from build123d import *

# Parameters (mm, degrees)
BOSS_EXTRUDE1_DEPTH     = 25.4
SKETCH2_R               = 3.175
BOSS_EXTRUDE3_DEPTH     = 3.81
BOSS_EXTRUDE4_START     = 3.81
SKETCH3_R               = 3.175
BOSS_EXTRUDE4_DEPTH     = 3.81
SKETCH4_W               = 19.976191583
SKETCH4_H               = 93.98
BOSS_EXTRUDE5_DEPTH     = 5.08
CUT_EXTRUDE1_DEPTH      = 5.08
CUT_EXTRUDE1_DEPTH_BACK = 381.820097899
SKETCH5_R               = 3.175


with BuildPart() as part:
    # Sketch1 → Boss-Extrude1 (new body)
    with BuildSketch(Plane.XY):
        with BuildLine():
            Line((-348.791316574, 206.904032246), (-347.931840304, 210.615824339))
            Line((-347.931840304, 210.615824339), (-357.71784023, 212.881801123))
            ThreePointArc((-357.71784023, 212.881801123), (-360.881852793, 214.462416261), (-362.982664296, 217.307747657))
            ThreePointArc((-362.982664296, 217.307747657), (-363.332122594, 222.183147168), (-360.629697113, 226.256050065))
            ThreePointArc((-360.629697113, 226.256050065), (-361.446766946, 231.453900041), (-358.789055407, 235.995025106))
            Line((-358.789055407, 235.995025106), (-363.476973871, 237.08052628))
            Line((-363.476973871, 237.08052628), (-369.361521397, 211.667123083))
            Line((-369.361521397, 211.667123083), (-348.791316574, 206.904032246))
        make_face()
    extrude(amount=-BOSS_EXTRUDE1_DEPTH)

    # Sketch2 → Boss-Extrude3 (add)
    # profile 1 of 2: a face of its own
    with BuildSketch(Plane(origin=(0, 0, -25.4), x_dir=(-1, 0, 0), z_dir=(0, 0, -1))):
        with BuildLine():
            Line((342.906769048, 232.317435443), (358.789055407, 235.995025106))
            ThreePointArc((358.789055407, 235.995025106), (361.446766946, 231.453900041), (360.629697113, 226.256050065))
            ThreePointArc((360.629697113, 226.256050065), (363.40772554, 218.647103628), (357.71784023, 212.881801123))
            Line((357.71784023, 212.881801123), (347.931840304, 210.615824339))
            Line((347.931840304, 210.615824339), (342.906769048, 232.317435443))
        make_face()
        with Locations(Location((353.754071424, 230, 0), (0, 0, 180))):
            Circle(SKETCH2_R, mode=Mode.SUBTRACT)
        with Locations(Location((356.009914651, 220.257763535, 0), (0, 0, 180))):
            Circle(SKETCH2_R, mode=Mode.SUBTRACT)
    # profile 2 of 2: a face of its own
    with BuildSketch(Plane(origin=(0, 0, -25.4), x_dir=(-1, 0, 0), z_dir=(0, 0, -1))):
        with BuildLine():
            ThreePointArc((360.629697113, 226.256050065), (363.40772554, 218.647103628), (357.71784023, 212.881801123))
            Line((357.71784023, 212.881801123), (347.931840304, 210.615824339))
            Line((347.931840304, 210.615824339), (348.791316574, 206.904032246))
            Line((348.791316574, 206.904032246), (369.361521397, 211.667123083))
            Line((369.361521397, 211.667123083), (363.476973871, 237.08052628))
            Line((363.476973871, 237.08052628), (358.789055407, 235.995025106))
            ThreePointArc((358.789055407, 235.995025106), (361.446766946, 231.453900041), (360.629697113, 226.256050065))
        make_face()
    extrude(amount=BOSS_EXTRUDE3_DEPTH)

    # Sketch3 → Boss-Extrude4 (add)
    # profile 1 of 2: a face of its own
    with BuildSketch(Plane.XY.offset(BOSS_EXTRUDE4_START)):
        with BuildLine():
            Line((-342.906769048, 232.317435443), (-358.789055407, 235.995025106))
            ThreePointArc((-358.789055407, 235.995025106), (-361.446766946, 231.453900041), (-360.629697113, 226.256050065))
            ThreePointArc((-360.629697113, 226.256050065), (-363.40772554, 218.647103628), (-357.71784023, 212.881801123))
            Line((-357.71784023, 212.881801123), (-347.931840304, 210.615824339))
            Line((-347.931840304, 210.615824339), (-342.906769048, 232.317435443))
        make_face()
        with Locations((-356.009914651, 220.257763535)):
            Circle(SKETCH3_R, mode=Mode.SUBTRACT)
        with Locations((-353.754071424, 230)):
            Circle(SKETCH3_R, mode=Mode.SUBTRACT)
    # profile 2 of 2: a face of its own
    with BuildSketch(Plane.XY.offset(BOSS_EXTRUDE4_START)):
        with BuildLine():
            Line((-347.931840304, 210.615824339), (-357.71784023, 212.881801123))
            ThreePointArc((-357.71784023, 212.881801123), (-363.40772554, 218.647103628), (-360.629697113, 226.256050065))
            ThreePointArc((-360.629697113, 226.256050065), (-361.446766946, 231.453900041), (-358.789055407, 235.995025106))
            Line((-358.789055407, 235.995025106), (-363.476973871, 237.08052628))
            Line((-363.476973871, 237.08052628), (-369.361521397, 211.667123083))
            Line((-369.361521397, 211.667123083), (-348.791316574, 206.904032246))
            Line((-348.791316574, 206.904032246), (-347.931840304, 210.615824339))
        make_face()
    extrude(amount=-BOSS_EXTRUDE4_DEPTH)

    # Sketch4 → Boss-Extrude5 (add)
    with BuildSketch(Plane(origin=(0, 211.667123083, 0), x_dir=(1, 0, 0), z_dir=(0, 1, 0))):
        with Locations((-365.660654241, 10.16)):
            Rectangle(SKETCH4_W, SKETCH4_H)
    extrude(amount=-BOSS_EXTRUDE5_DEPTH)

    # Sketch5 → Cut-Extrude1 (cut, two sides: drawn at the far end of the back side and taken through both)
    with BuildSketch(Plane(origin=(0, 211.667123083, 0), x_dir=(1, 0, 0), z_dir=(0, 1, 0)).offset(-CUT_EXTRUDE1_DEPTH_BACK)):
        with Locations(Location((-366.758750033, 43.909082713, 0), (0, 0, 270))):
            Circle(SKETCH5_R)
        with Locations(Location((-366.758750033, -31.331908304, 0), (0, 0, 270))):
            Circle(SKETCH5_R)
    extrude(amount=CUT_EXTRUDE1_DEPTH + CUT_EXTRUDE1_DEPTH_BACK, mode=Mode.SUBTRACT)


solid = part.part
Can you work these out from the model? Positions are in its coordinate system, mm. A direction names the side the tool comes from. Round coordinates to 2 decimals unless told otherwise and drop trailing zeros. Loops run counter-clockwise (first coordinate to the right, second up) from the corner with the lowest first, then second, coordinate; pieces in that order, holes last. Notation, with made-up numbers: (45.5, 28) - (52.5, 28) arc R8 ccw to (52.5, 33) - close; hole circle Ø3 at (46, 74.25). An arc over 180 degrees is marked (long way). Use CSV: the item, a comma, the result in double quotes. Start each with the question number.
1) For faces 1 (the flat face through (-352.28, 207.71, -12.47)), 2 (the flat face through (-353, 223, -25.4)), 3 (the flat face through (-352.756, 211.733, -12.522)), which set-ups out of +Z, -Z, +X, -X, +Y, -Y let a thin tool reach every point of the face, with its end or its side?
2) If we section it at C-C on y = 235: Write out the boundary of the cut face in (x, z), plus the area to 3 significant figures.
3) If we section it at A-A on z = -10: Write out the boundary of the cut face in (x, y), plus the area to 3 significant figures.
4) If we section it at B-B on y = 219: Write out the boundary of the cut face in (x, z), plus the area to 3 significant figures.
5) For pin 1 Ø10 at (x, z) = (-366.76, 31.33) entering from +Y; pin 2 Ø13 at (x, y) = (-362, 216.5) entering from +Z; pin 3 Ø4 at (x, y) = (-353.75, 230) entering from -Z; pin 4 Ø16.5 at (x, y) = (-357.5, 222.5) entering from -Z, each with a flat end and sliding along its axis, tell me the tip position at first contact or that it passes through.
6) If we section it at D-D on y = 230: Write out the boundary of the cut face in (x, z).
7) We'd pull the mould along X, two halves only. Please class faces 4 (the flat face through (-353, 222, 3.81)), 5 (the flat face through (-375.649, 209, -10)), 6 (the cylindrical face through (-369.858, 209.092, 30.644)): released by +X, released by -X, zero draft, split by the parting line, or undercut.
8) Please list where these lines run through material, in increasing order: probe 1 along Y at (x, z) = (-353.5, 1); probe 2 along Z at (x, y) = (-365.5, 208.5); probe 3 along Z at (x, y) = (-358, 233.5). Write a range as [from, to].
Geometry results:
1,face 1,"+Z, -Z, -Y"
1,face 2,"+X"
1,face 3,"+X, +Y"
2,outline,"(-363.96, -29.21) - (-354.49, -29.21) - (-354.49, -25.4) - (-359.78, -25.4) - (-359.78, 0) - (-354.49, 0) - (-354.49, 3.81) - (-363.96, 3.81) - close"
2,area,"178 mm2"
3,outline,"(-375.65, 206.59) - (-355.67, 206.59) - (-355.67, 208.5) - (-348.79, 206.9) - (-347.93, 210.62) - (-357.72, 212.88) arc R7.57 cw to (-360.63, 226.26) arc R7.83 cw to (-358.79, 236) - (-363.48, 237.08) - (-369.36, 211.67) - (-375.65, 211.67) - close"
3,area,"256 mm2"
4,outline,"(-367.66, -29.21) - (-358.93, -29.21) - (-358.93, -25.4) - (-363.48, -25.4) - (-363.48, 0) - (-358.93, 0) - (-358.93, 3.81) - (-367.66, 3.81) - close; (-353.09, -29.21) - (-345.99, -29.21) - (-345.99, -25.4) - (-353.09, -25.4) - close; (-353.09, 0) - (-345.99, 0) - (-345.99, 3.81) - (-353.09, 3.81) - close"
4,area,"227 mm2"
5,pin 1,"stops at y = 211.67"
5,pin 2,"stops at z = 36.83"
5,pin 3,"passes through"
5,pin 4,"stops at z = -29.21"
6,outline,"(-365.12, -29.21) - (-356.93, -29.21) - (-356.93, -25.4) - (-361.58, -25.4) - (-361.58, 0) - (-356.93, 0) - (-356.93, 3.81) - (-365.12, 3.81) - close; (-350.58, -29.21) - (-343.44, -29.21) - (-343.44, -25.4) - (-350.58, -25.4) - close; (-350.58, 0) - (-343.44, 0) - (-343.44, 3.81) - (-350.58, 3.81) - close"
7,face 4,"zero draft"
7,face 5,"released by -X"
7,face 6,"undercut"
8,probe 1,"y = [207.99, 218.31], [222.2, 226.84], [233.16, 234.77]"
8,probe 2,"z = [-57.15, -46.82], [-40.99, 28.42], [34.25, 36.83]"
8,probe 3,"z = [-29.21, -25.4], [0, 3.81]"
